Design review of the part built by this model. Coordinates are the model's own, in mm. A direction names the side the tool comes from. Round coordinates to 2 decimals unless told otherwise and drop trailing zeros. Order: outer loops, then holes, each group sorted by start corner. A loop starts at its lowest first (then second) coordinate and runs counter-clockwise, first axis right, second up. Notation, with made-up numbers: M 66,14 L 79,14 A25 ccw 79,28 Z; hole C 34.25,64 d4. An arc over 180 degrees is marked long. Use a Markdown table: item, result. Add a question column.
(1) Take a section at B-B (y = -1.7). Write out the cut boundary in (x, z) (1 decimal), then the cut area to 3 significant figures.
(2) Machinability: for faces 1 (the face through (2.66, -1.84, -19.7)), 2 (the face through (-3.47, -1.84, -16.73)), which of the approach directions +Z, -Z, +X, -X, +Y, -Y give a long, thin tool a straight path to every point of the face, cutting with its end or side? Answer none if there is none.
(3) Take a section at D-D (z = 10). Write out the cut boundary in (x, y).
(4) Take a section at C-C (x = 5). Write out the cut boundary in (y, z).
(5) For pin 1 (2 mm diameter, centred on x = -20.5, y = -2.5, fed in from -Z); pin 2 (1 mm diameter, centred on y = -2.5, z = 8, fed in from -X); pin 3 (1 mm diameter, centred on y = -1, z = -11.5, fed in from -X); pin 4 (17.5 mm diameter, centred on x = 13.59, z = -20.68, fed in from +Y), all flat-tipped, find the tip position at first contact; note any pin that passes through.
(6) To check wall thickness, follow probe 1 along X at (y, z) = (-1, -13); probe 2 along X at (y, z) = (-3.15, 3); probe 3 along Z at (x, y) = (9.5, -1). State the ranges of each line that lie inside material, in increasing order. Write a range as from..to.
(7) Take a section at A-A (z = -1). Write out the cut boundary in (x, y).
(8) The part is to be moulded in two halves that separate along Z. For faces 3 (the face through (-9.41, -1.84, -10.11)), 4 (the face through (5.545, -1.844, -4.303)), 5 (the face through (-14, 0, -8)), 6 (the face through (-25.272, -1.844, 3.299)), say which applies: released by +Z, released by -Z, zero draft, split by the parting line, or undercut.
```python
from build123d import *

# Parameters (mm, degrees)
F0_R     = 4.1529
F1_DEPTH = 3.74112
F2_R     = 5.3975
F3_DEPTH = 25.4


with BuildPart() as f1:
    # F0 (on Front) → F1 (new body)
    with BuildSketch(Plane.XZ):
        Polygon((-1.106079, -16.707432), (6.419018, -7.234566), (4.326342, -5.488987), (-3.466987, -14.831964), align=None)
        Polygon((-20.885671, -3.838109), (-22.564381, 8.295304), (-26.106817, 9.332149), (-24.413652, -2.905742), align=None)
        with BuildLine():
            ThreePointArc((13.531608, -13.167445), (15.255443, -13.354337), (16.890565, -13.931319))
            Line((16.890565, -13.931319), (-6.122345, 5.599705))
            Line((-6.122345, 5.599705), (-40.019221, 15.604509))
            Line((-40.019221, 15.604509), (-43.453703, 0))
            Line((-43.453703, 0), (-15.522079, -7.155403))
            Line((-15.522079, -7.155403), (8.91424, -26.567232))
            ThreePointArc((8.91424, -26.567232), (7.30033, -24.797842), (6.325001, -22.610565))
            Line((6.325001, -22.610565), (-1.106079, -16.707432))
            Line((-1.106079, -16.707432), (-3.466987, -14.831964))
            Line((-3.466987, -14.831964), (-15.522079, -5.255588))
            Line((-15.522079, -5.255588), (-20.885671, -3.838109))
            Line((-20.885671, -3.838109), (-24.413652, -2.905742))
            Line((-24.413652, -2.905742), (-41.059079, 1.493276))
            Line((-41.059079, 1.493276), (-38.533263, 12.969277))
            Line((-38.533263, 12.969277), (-26.106817, 9.332149))
            Line((-26.106817, 9.332149), (-22.564381, 8.295304))
            Line((-22.564381, 8.295304), (-6.595499, 3.621332))
            Line((-6.595499, 3.621332), (4.326342, -5.488987))
            Line((4.326342, -5.488987), (6.419018, -7.234566))
            Line((6.419018, -7.234566), (13.531608, -13.167445))
        make_face()
        with BuildLine():
            ThreePointArc((8.91424, -26.567232), (16.856094, -27.450659), (21.104277, -20.682615))
            ThreePointArc((21.104277, -20.682615), (19.964406, -16.703439), (16.890565, -13.931319))
            ThreePointArc((16.890565, -13.931319), (15.255443, -13.354337), (13.531608, -13.167445))
            ThreePointArc((13.531608, -13.167445), (7.614526, -16.123223), (6.325001, -22.610565))
            ThreePointArc((6.325001, -22.610565), (7.30033, -24.797842), (8.91424, -26.567232))
        make_face()
        with Locations((13.588889, -20.682615)):
            Circle(F0_R, mode=Mode.SUBTRACT)
        with Locations((13.588889, -20.682615)):
            Circle(F0_R)
    extrude(amount=F1_DEPTH)

    # F2 (on face) → F3 (cut)
    with BuildSketch(Plane(origin=(0, 0, 0), x_dir=(-1, 0, 0), z_dir=(0, 1, 0))):
        with Locations((-13.588889, -20.682615)):
            Circle(F2_R)
    extrude(amount=-F3_DEPTH, mode=Mode.SUBTRACT)


solid = f1.part
```
Verdict:
| question | item | result |
|---|---|---|
| 1 | outline | M -43.5,0 L -15.5,-7.2 L 8.9,-26.6 A7.5 ccw long 16.9,-13.9 L -6.1,5.6 L -40,15.6 Z; hole M -41.1,1.5 L -24.4,-2.9 L -26.1,9.3 L -38.5,13 Z; hole M -22.6,8.3 L -20.9,-3.8 L -15.5,-5.3 L -3.5,-14.8 L 4.3,-5.5 L -6.6,3.6 Z; hole M -1.1,-16.7 L 6.3,-22.6 A7.5 cw 13.5,-13.2 L 6.4,-7.2 Z; hole C 13.6,-20.7 d10.8 |
| 1 | area | 405 mm^2 |
| 2 | face 1 | +Y, -Y |
| 2 | face 2 | -Z, -X, +Y, -Y |
| 3 | outline | M -41.25,-3.74 L -39.19,-3.74 L -39.19,0 L -41.25,0 Z; M -28.39,-3.74 L -21.03,-3.74 L -21.03,0 L -28.39,0 Z |
| 4 | outline | M -3.74,-23.46 L 0,-23.46 L 0,-21.56 L -3.74,-21.56 Z; M -3.74,-9.02 L 0,-9.02 L 0,-3.84 L -3.74,-3.84 Z |
| 5 | pin 1 | stops at z = -6.14 |
| 5 | pin 2 | stops at x = -41.8 |
| 5 | pin 3 | stops at x = -10.68 |
| 5 | pin 4 | stops at y = 0 |
| 6 | probe 1 | x = -8.16..-5.77, -1.94..1.84, 13.33..15.79 |
| 6 | probe 2 | x = -42.79..-40.73, -25.23..-21.83, -5.85..-3.06 |
| 6 | probe 3 | z = -26.99..-24.21, -17.16..-14.38, -9.8..-7.66 |
| 7 | outline | M -39.55,-3.74 L -31.62,-3.74 L -31.62,0 L -39.55,0 Z; M -24.68,-3.74 L -21.28,-3.74 L -21.28,0 L -24.68,0 Z; M -1.06,-3.74 L 1.65,-3.74 L 1.65,0 L -1.06,0 Z |
| 8 | face 3 | undercut |
| 8 | face 4 | released by +Z |
| 8 | face 5 | zero draft |
| 8 | face 6 | undercut |
